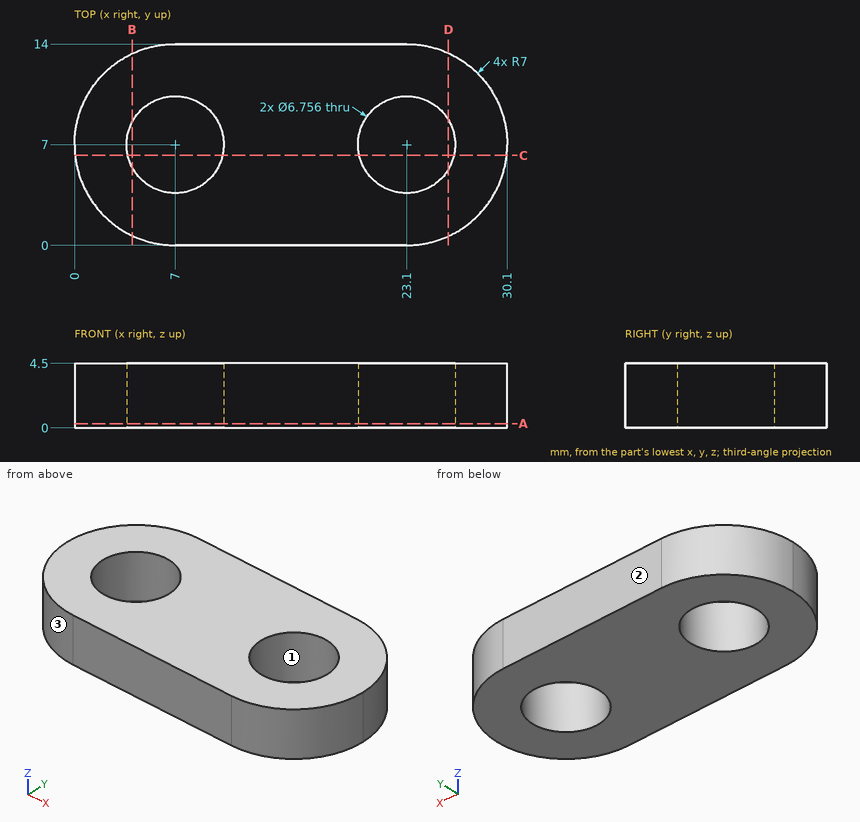
Print and shaded views of the part. All mm, measured from the part's lowest x, y and z. Coordinates: 2 decimals unless noted, no trailing zeros. Order: outer loops, then holes, each group sorted by start corner. A loop starts at its lowest first (then second) coordinate and runs counter-clockwise, first axis right, second up. Notation, with made-up numbers: M -40,-26 L 18,-26 A24 ccw 18,6 Z; hole C 54,74.5 d5. An arc over 180 degrees is marked long. One line per question, with ' | ' between items. Start each with the question number.
Q1. Probe L1, parallel to X at y = 7, z = 3.5; L2, parallel to Y at x = 23, z = 3.1; L3, parallel to X at y = 5.5, z = 2.4 (1 decimal). List the from-to ranges inside material, lowest first. Write a range as from..to.
Q2. Saw through at C-C (y = 6.25). List the corners of the cut face in (x, z).
Q3. Two-plate mould, pull along Y, no slides. Class the marked faces 1, 2 and 3: +Y half, -Y half, draft (parallel to the pull), parting line (faces both ways), or undercut.
Q4. Saw through at D-D (x = 26). List the corners of the cut face in (y, z).
Q5. Flat gauge pins, fed straight in: pin 1 Ø1.5 at (x, y) = (23, 6) entering from -Z; pin 2 Ø1 at (y, z) = (8, 2) entering from -X. Where does each tip first touch, or does it go through?
Q6. Saw through at A-A (z = 0.3). Count the separate pieces of the cut face and the enclosed holes in it, then the cut area to 3 significant figures.
Q7. Saw through at B-B (x = 4). List the corners of the cut face in (y, z) (1 decimal).
Check values:
1) L1: x = 0..3.62, 10.38..19.72, 26.48..30.1 | L2: y = 0..3.62, 10.38..14 | L3: x = 0.2..4, 10..20.1, 26.1..29.9
2) outline: M 0.04,0 L 3.71,0 L 3.71,4.5 L 0.04,4.5 Z; M 10.29,0 L 19.81,0 L 19.81,4.5 L 10.29,4.5 Z; M 26.39,0 L 30.06,0 L 30.06,4.5 L 26.39,4.5 Z
3) face 1: undercut | face 2: +Y half | face 3: -Y half
4) outline: M 0.63,0 L 5.27,0 L 5.27,4.5 L 0.63,4.5 Z; M 8.73,0 L 13.37,0 L 13.37,4.5 L 8.73,4.5 Z
5) pin 1: passes through | pin 2: stops at x = 0.02
6) separate pieces: 1 | enclosed holes: 2 | area: 308 mm2
7) outline: M 0.7,0 L 5.4,0 L 5.4,4.5 L 0.7,4.5 Z; M 8.6,0 L 13.3,0 L 13.3,4.5 L 8.6,4.5 Z
